For this review, take the finished solid that the model builds, in its own axes (mm). A direction names the side the tool comes from. Coordinates: 2 decimals unless noted, no trailing zeros. Order: outer loops, then holes, each group sorted by start corner. A loop starts at its lowest first (then second) coordinate and runs counter-clockwise, first axis right, second up. Notation, with made-up numbers: (64, 2) -> (78, 2) arc R33 ccw to (78, 38) -> close; hole circle Ø9 at (28.25, -29). An arc over 180 degrees is marked (long way). Return JSON: item names as keys, results as strings. Group by question number.
Item 1: Take a section at A-A (y = -7.5). Write out the cut boundary in (x, z).
Item 2: Take a section at D-D (x = 1.2). Write out the cut boundary in (y, z).
Item 3: Take a section at C-C (z = 0). Write out the cut boundary in (x, y).
Item 4: Take a section at B-B (z = -1.35). Write out the cut boundary in (x, y), then the cut area to 3 significant figures.
Item 5: Draft analysis for pull direction Y (two halves, no side actions). For faces 4 (the flat face through (-0.25, -12, 0)), 5 (the flat face through (1, 0, -1)), 6 (the cylindrical face through (-0.004, -12.459, 1.515)), state which applies: +Y half, -Y half, draft (parallel to the pull), parting line (faces both ways), or undercut.
Item 6: Insertion check: pin 1 (2 mm diameter, centred on y = -5.5, z = 0.5, fed in from -X); pin 2 (1.3 mm diameter, centred on y = -11, z = 0, fed in from +X); pin 3 (2 mm diameter, centred on y = -11, z = -0.5, fed in from -X). Each pin has a flat end and moves straight along its axis. Give the tip position at first contact, or say it passes through.
Item 7: For line 1 along X through (y, z) = (0.15, 0); line 2 along Y through (x, z) = (-0.95, 1.9); line 3 along X through (y, z) = (-7.25, 1.3), list the stretches that pass through material, from the lowest coordinate up.
Item 8: Machinability: for faces 1 (the cylindrical face through (-0.004, -12.475, -1.499)), 2 (the flat face through (-0.934, -5.282, 0.825)), 3 (the flat face through (0.25, -12, 0)), which of the approach directions +Z, -Z, +X, -X, +Y, -Y give a long, thin tool a straight path to every point of the face, cutting with its end or side? Answer none if there is none.
```python
from build123d import *

# Parameters (mm, degrees)
ESBO_O1_R                = 1.05
RESSALTO_EXTRUS_O1_DEPTH = 0.25
RESSALTO_EXTRUS_O2_DEPTH = 1.8
FILETE1_R                = 1
RESSALTO_EXTRUS_O4_DEPTH = 2
CORTE_EXTRUS_O6_DEPTH    = 5
ESBO_O5_R                = 1.05
RESSALTO_EXTRUS_O3_DEPTH = 0.7
CORTE_EXTRUS_O1_DEPTH    = 5
CORTE_EXTRUS_O2_DEPTH    = 15


with BuildPart() as part:
    # Esboço1 → Ressalto-extrusão1 (new body)
    with BuildSketch(Plane(origin=(0, 0, 0), x_dir=(1, 0, 0), z_dir=(0, 1, 0))):
        with BuildLine():
            Line((2.079062289, 1.8), (14, 1.8))
            ThreePointArc((14, 1.8), (14.707106781, 1.507106781), (15, 0.8))
            Line((15, 0.8), (15, -0.8))
            ThreePointArc((15, -0.8), (14.707106781, -1.507106781), (14, -1.8))
            Line((14, -1.8), (2.079062289, -1.8))
            ThreePointArc((2.079062289, -1.8), (0, -2.75), (-2.079062289, -1.8))
            Line((-2.079062289, -1.8), (-14, -1.8))
            ThreePointArc((-14, -1.8), (-14.707106781, -1.507106781), (-15, -0.8))
            Line((-15, -0.8), (-15, 0.8))
            ThreePointArc((-15, 0.8), (-14.707106781, 1.507106781), (-14, 1.8))
            Line((-14, 1.8), (-2.079062289, 1.8))
            ThreePointArc((-2.079062289, 1.8), (0, 2.75), (2.079062289, 1.8))
        make_face()
        with Locations(Location((0, 0, 0), (0, 0, 270))):
            Circle(ESBO_O1_R, mode=Mode.SUBTRACT)
        with BuildLine():
            Line((4.978511643, 0.549893952), (12.857420168, 0.15))
            ThreePointArc((12.857420168, 0.15), (13, 0), (12.857420168, -0.15))
            Line((12.857420168, -0.15), (4.978511643, -0.549893952))
            ThreePointArc((4.978511643, -0.549893952), (4.4, 0), (4.978511643, 0.549893952))
        make_face(mode=Mode.SUBTRACT)
        with BuildLine():
            Line((-12.857420168, -0.15), (-4.978511643, -0.549893952))
            ThreePointArc((-4.978511643, -0.549893952), (-4.4, 0), (-4.978511643, 0.549893952))
            Line((-4.978511643, 0.549893952), (-12.857420168, 0.15))
            ThreePointArc((-12.857420168, 0.15), (-13, 0), (-12.857420168, -0.15))
        make_face(mode=Mode.SUBTRACT)
    extrude(amount=RESSALTO_EXTRUS_O1_DEPTH)


with BuildPart() as body_2:
    # Esboço4 → Ressalto-extrusão2 (new, symmetric)
    with BuildSketch(Plane.XY):
        with BuildLine():
            Line((0, -10.226584075), (0, -12.76))
            Line((0, -12.76), (-0.25, -12.76))
            Line((-0.25, -12.76), (-0.25, -10.25))
            Line((-0.25, -10.25), (-2.088694427, -0.52070389))
            ThreePointArc((-2.088694427, -0.52070389), (-1.950478535, 0.014754428), (-1.45, 0.25))
            Line((-1.45, 0.25), (-1.45, 0))
            ThreePointArc((-1.45, 0), (-1.757986791, -0.144766506), (-1.843042724, -0.474279317))
            Line((-1.843042724, -0.474279317), (0, -10.226584075))
        make_face()
    extrude(amount=RESSALTO_EXTRUS_O2_DEPTH, both=True)

    # Filete1
    filete1_edges = [body_2.edges().sort_by_distance(p)[0] for p in [
        (-0.125, -12.76, 1.8),
        (-0.125, -12.76, -1.8),
    ]]
    fillet(filete1_edges, radius=FILETE1_R)


with BuildPart() as body_3:
    # Esboço16 → Ressalto-extrusão4 (new, symmetric)
    with BuildSketch(Plane.ZY.offset(0.25)):
        with BuildLine():
            Line((0.15, -10.61), (0.549854071, -2.738494336))
            ThreePointArc((0.549854071, -2.738494336), (0, -2.16), (-0.549854071, -2.738494336))
            Line((-0.549854071, -2.738494336), (-0.15, -10.61))
            ThreePointArc((-0.15, -10.61), (0, -10.76), (0.15, -10.61))
        make_face()
    extrude(amount=RESSALTO_EXTRUS_O4_DEPTH, both=True)

    # Esboço17 → Corte-extrusão6 (cut, symmetric)
    with BuildSketch(Plane(origin=(-2.111680199, -0.399076621, 0), x_dir=(0, 0, 1), z_dir=(-0.9826068107203668, -0.18569829166136476, 0))):
        with BuildLine():
            Line((-0.55, -2.513436729), (-0.175, -10.025295237))
            Line((-0.175, -10.025295237), (-1.291075027, -10.025295237))
            Line((-1.291075027, -10.025295237), (-1.291075027, -1.561962936))
            Line((-1.291075027, -1.561962936), (1.201455883, -1.561962936))
            Line((1.201455883, -1.561962936), (1.201455883, -10.025295237))
            Line((1.201455883, -10.025295237), (0.175, -10.025295237))
            Line((0.175, -10.025295237), (0.55, -2.513436729))
            ThreePointArc((0.55, -2.513436729), (0, -1.935295237), (-0.55, -2.513436729))
        make_face()
    extrude(amount=CORTE_EXTRUS_O6_DEPTH, both=True, mode=Mode.SUBTRACT)


with BuildPart() as body_2_1:
    add(body_2.part)

    # Combinar2: cut body 3
    add(body_3.part, mode=Mode.SUBTRACT)


with BuildPart() as body_3_2:
    # Espelhar1: mirrored copy
    add(body_2_1.part.mirror(Plane(origin=(0, 0, 0), x_dir=(0, 0, 1), z_dir=(1, 0, 0))))


with BuildPart() as body_4:
    # Esboço5 → Ressalto-extrusão3 (new body)
    with BuildSketch(Plane(origin=(0, 0.25, 0), x_dir=(1, 0, 0), z_dir=(0, 1, 0))):
        with BuildLine():
            Line((-2.1, 1.852025918), (-2.1, -1.852025918))
            ThreePointArc((-2.1, -1.852025918), (0, -2.8), (2.1, -1.852025918))
            Line((2.1, -1.852025918), (2.1, 1.852025918))
            ThreePointArc((2.1, 1.852025918), (0, 2.8), (-2.1, 1.852025918))
        make_face()
        with Locations(Location((0, 0, 0), (0, 0, 270))):
            Circle(ESBO_O5_R, mode=Mode.SUBTRACT)
    extrude(amount=-RESSALTO_EXTRUS_O3_DEPTH)

    # Esboço6 → Corte-extrusão1 (cut, symmetric)
    with BuildSketch(Plane.XY):
        with BuildLine():
            Line((-1.45, 0.25), (-1.45, 0.597201145))
            Line((-1.45, 0.597201145), (-2.428627535, 0.597201145))
            Line((-2.428627535, 0.597201145), (-2.428627535, -0.52070389))
            Line((-2.428627535, -0.52070389), (-2.088694427, -0.52070389))
            ThreePointArc((-2.088694427, -0.52070389), (-1.950478535, 0.014754428), (-1.45, 0.25))
        make_face()
        with BuildLine():
            Line((1.45, 0.25), (1.45, 0.729701811))
            Line((1.45, 0.729701811), (2.688745217, 0.729701811))
            Line((2.688745217, 0.729701811), (2.688745217, -0.52070389))
            Line((2.688745217, -0.52070389), (2.088694427, -0.52070389))
            ThreePointArc((2.088694427, -0.52070389), (1.950478535, 0.014754428), (1.45, 0.25))
        make_face()
        with BuildLine():
            Line((-1.45, 0), (1.45, 0))
            ThreePointArc((1.45, 0), (1.757986791, -0.144766506), (1.843042724, -0.474279317))
            Line((1.843042724, -0.474279317), (-1.843042724, -0.474279317))
            ThreePointArc((-1.843042724, -0.474279317), (-1.757986791, -0.144766506), (-1.45, 0))
        make_face()
    extrude(amount=CORTE_EXTRUS_O1_DEPTH, both=True, mode=Mode.SUBTRACT)

    # Combinar1: union body 3 2, body 2
    add(body_3_2.part)
    add(body_2_1.part)

    # Esboço7 → Corte-extrusão2 (cut, symmetric)
    with BuildSketch(Plane(origin=(0, 0, 0), x_dir=(0, 0, -1), z_dir=(1, 0, 0))):
        with BuildLine():
            Line((2.395307913, 0), (3.16000301, 0))
            Line((3.16000301, 0), (3.16000301, -0.618768346))
            Line((3.16000301, -0.618768346), (1.8, -0.618768346))
            Line((1.8, -0.618768346), (1.8, -0.45))
            ThreePointArc((1.8, -0.45), (2.022182093, -0.125157783), (2.395307913, 0))
        make_face()
        with BuildLine():
            Line((-1.8, -0.45), (-1.8, -0.594962274))
            Line((-1.8, -0.594962274), (-2.989404484, -0.594962274))
            Line((-2.989404484, -0.594962274), (-2.989404484, 0))
            Line((-2.989404484, 0), (-2.395307913, 0))
            ThreePointArc((-2.395307913, 0), (-2.022182093, -0.125157783), (-1.8, -0.45))
        make_face()
    extrude(amount=CORTE_EXTRUS_O2_DEPTH, both=True, mode=Mode.SUBTRACT)


solid = body_4.part
```
Findings below:
{
 "1": {"outline": "(-0.77, -1.8) -> (-0.52, -1.8) -> (-0.52, -0.31) -> (-0.77, -0.31) -> close; (-0.77, 0.31) -> (-0.52, 0.31) -> (-0.52, 1.8) -> (-0.77, 1.8) -> close; (0.52, -1.8) -> (0.77, -1.8) -> (0.77, -0.31) -> (0.52, -0.31) -> close; (0.52, 0.31) -> (0.77, 0.31) -> (0.77, 1.8) -> (0.52, 1.8) -> close"},
 "2": {"outline": "(-5.22, -1.8) -> (-3.88, -1.8) -> (-3.88, -0.49) -> (-5.22, -0.42) -> close; (-5.22, 0.42) -> (-3.88, 0.49) -> (-3.88, 1.8) -> (-5.22, 1.8) -> close; (0, -2.53) -> (0.25, -2.53) -> (0.25, 2.53) -> (0, 2.53) -> close"},
 "3": {"outline": "(-2.09, -0.52) -> (-1.75, -2.3) -> (-1.51, -2.25) -> (-1.84, -0.47) arc R0.4 cw to (-1.45, 0) -> (-1.05, 0) -> (-1.05, 0.25) -> (-1.45, 0.25) arc R0.65 ccw to start; (-0.25, -12.76) -> (0.25, -12.76) -> (0.25, -10.76) -> (-0.25, -10.76) -> close; (1.05, 0) -> (1.45, 0) arc R0.4 cw to (1.84, -0.47) -> (1.51, -2.25) -> (1.75, -2.3) -> (2.09, -0.52) arc R0.65 ccw to (1.45, 0.25) -> (1.05, 0.25) -> close"},
 "4": {"outline": "(-2.09, -0.52) -> (-0.25, -10.25) -> (-0.25, -12.6) -> (0.25, -12.6) -> (0.25, -10.25) -> (2.09, -0.52) arc R0.65 ccw to (1.45, 0.25) -> (-1.45, 0.25) arc R0.65 ccw to start; hole (-1.84, -0.47) -> (0, -10.23) -> (1.84, -0.47) arc R0.4 ccw to (1.45, 0) -> (-1.45, 0) arc R0.4 ccw to start", "area": "7.32 mm2"},
 "5": {"face 4": "draft", "face 5": "undercut", "face 6": "-Y half"},
 "6": {"pin 1": "stops at x = -1.34", "pin 2": "stops at x = 0.25", "pin 3": "stops at x = -0.3"},
 "7": {"line 1": "x = -1.8 to -1.05, 1.05 to 1.8", "line 2": "y = 0 to 0.25", "line 3": "x = -0.82 to -0.56, 0.56 to 0.82"},
 "8": {"face 1": "-Z, +X, -X, -Y", "face 2": "+Z, -Z", "face 3": "+Z, -Z, +X, -Y"}
}
